```python
from build123d import *

# Parameters (mm, degrees)
F1_DEPTH = 12.5
F2_R     = 2.125
F3_DEPTH = 5.001
F4_R     = 2.125
F5_DEPTH = 5.001
F6_R     = 2.5
F7_R     = 3.5
F8_DEPTH = 20.001


with BuildPart() as f1:
    # F0 (on Right) → F1 (new body, symmetric)
    with BuildSketch(Plane.YZ):
        Polygon((5, 25), (0, 25), (0, 0), (15, 0), (15, 5), (10, 5), (5, 10), align=None)
    extrude(amount=F1_DEPTH, both=True)

    # F2 (on face) → F3 (cut, through all)
    with BuildSketch(Plane.XY.offset(5)):
        with Locations((0, 10)):
            Circle(F2_R)
    extrude(amount=-F3_DEPTH, mode=Mode.SUBTRACT)

    # F4 (on face) → F5 (cut, through all)
    with BuildSketch(Plane(origin=(0, 5, 0), x_dir=(-1, 0, 0), z_dir=(0, 1, 0))):
        with Locations((0, 17.5)):
            Circle(F4_R)
    extrude(amount=-F5_DEPTH, mode=Mode.SUBTRACT)

    # F6
    f6_edges = [f1.edges().sort_by_distance(p)[0] for p in [
        (0, 15, 5),
        (0, 5, 25),
    ]]
    fillet(f6_edges, radius=F6_R)

    # F7 (on face) → F8 (cut, through all)
    with BuildSketch(Plane(origin=(0, 0, 5), x_dir=(1, 0, 0), z_dir=(0, 0, -1))):
        with Locations((0, -10)):
            Circle(F7_R)
    extrude(amount=-F8_DEPTH, mode=Mode.SUBTRACT)


solid = f1.part
```
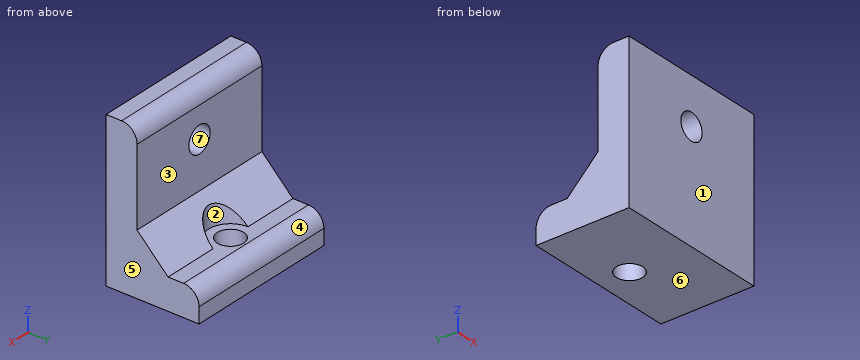
Read the model definition and answer for the solid it produces. Units are mm, in the model's axes. Face numbers are marked on the shaded views. A direction names the side the tool comes from. Give positions to 0.01 mm unless a question says otherwise; leave off trailing zeros. Order: outer loops, then holes, each group sorted by start corner. A loop starts at its lowest first (then second) coordinate and runs counter-clockwise, first axis right, second up. Notation, with made-up numbers: (59.5, -30.75) -> (91.5, -30.75) arc R15 cw to (91.5, -13.75) -> close; hole circle Ø6 at (42, 83.5). An arc over 180 degrees is marked (long way). One line per item, written item: value. Start each with the question number.
(1) The part is cut by section D-D (x = -8). Determine the outline of the cut face in (y, z).
(2) Flat-ended cylindrical pins translate along their axes: P1, Ø6, axis at x = -0.5, z = 16, coming from the +Y side; P2, Ø3, axis at x = -4, y = 9.5, coming from the +Z side; P3, Ø1.5, axis at x = 6.5, y = 5.5, coming from the +Z side. Find the tip coordinate at first contact, or state that the pin passes through.
(3) The part is cut by section C-C (y = 1.5). Determine the outline of the cut face in (x, z) (3 decimals), and give its area (3 significant figures).
(4) A tool of negligible diameter and unlimited length cuts with its end or side. For the marked faces 1, 2 and 3, from which of +Z, -Z, +X, -X, +Y, -Y can it reach the whole face along a straight path? Write none if from no direction.
(5) The part is cut by section A-A (z = 17.5). Determine the outline of the cut face in (x, y) (3 decimals).
(6) The part is cut by section B-B (x = 0). Determine the outline of the cut face in (y, z) (3 decimals).
(7) Straight lines are drawn through the part: L1, parallel to Y at x = 0, z = 2.1 (3 decimals); L2, parallel to Z at x = 0, y = 2.45 (3 decimals); L3, parallel to Y at x = -8.75, z = 18.5. For each, find the intervals that lie inside material, in ascending order.
(8) For a pull along Z with two mould halves and no side action, classify the marked faces 4, 5, 6 and 7 as released by +Z, released by -Z, zero draft, split by the parting line, or undercut.
Taken from the geometry:
1. outline: (0, 0) -> (15, 0) -> (15, 2.5) arc R2.5 ccw to (12.5, 5) -> (10, 5) -> (5, 10) -> (5, 22.5) arc R2.5 ccw to (2.5, 25) -> (0, 25) -> close
2. P1: y = 5
2. P2: z = 7
2. P3: z = 23.59
3. outline: (-12.5, 0) -> (12.5, 0) -> (12.5, 25) -> (-12.5, 25) -> close; hole circle Ø4.25 at (0, 17.5)
3. area: 611 mm^2
4. face 1: +Z, -Z, +X, -X, -Y
4. face 2: +Z, +Y
4. face 3: +Z, +X, -X, +Y
5. outline: (-12.5, 0) -> (-2.125, 0) -> (-2.125, 5) -> (-12.5, 5) -> close; (2.125, 0) -> (12.5, 0) -> (12.5, 5) -> (2.125, 5) -> close
6. outline: (0, 0) -> (7.875, 0) -> (7.875, 5) -> (6.5, 5) -> (6.5, 8.5) -> (5, 10) -> (5, 15.375) -> (0, 15.375) -> close; (0, 19.625) -> (5, 19.625) -> (5, 22.5) arc R2.5 ccw to (2.5, 25) -> (0, 25) -> close; (12.125, 0) -> (15, 0) -> (15, 2.5) arc R2.5 ccw to (12.5, 5) -> (12.125, 5) -> close
7. L1: 0 to 7.875, 12.125 to 15
7. L2: 0 to 15.375, 19.625 to 25
7. L3: 0 to 5
8. face 4: released by +Z
8. face 5: zero draft
8. face 6: released by -Z
8. face 7: undercut
